```python
from build123d import *

# Parameters (mm, degrees)
CROQUIS2_W              = 135
CROQUIS2_H              = 90
CROQUIS2_R              = 6
SALIENTE_EXTRUIR1_DEPTH = 10
CROQUIS3_W              = 75
CROQUIS3_H              = 90
SALIENTE_EXTRUIR2_DEPTH = 10
CROQUIS4_W              = 55
CROQUIS4_H              = 20
CORTAR_EXTRUIR1_DEPTH   = 91
SALIENTE_EXTRUIR3_DEPTH = 6
CROQUIS11_R             = 10
SALIENTE_EXTRUIR4_DEPTH = 37.5
SALIENTE_EXTRUIR5_DEPTH = 3


with BuildPart() as part:
    # Croquis2 → Saliente-Extruir1 (new body)
    with BuildSketch(Plane(origin=(0, 0, 0), x_dir=(1, 0, 0), z_dir=(0, 1, 0))):
        Rectangle(CROQUIS2_W, CROQUIS2_H)
        with Locations((-53, -25)):
            Circle(CROQUIS2_R, mode=Mode.SUBTRACT)
        with Locations((53, -25)):
            Circle(CROQUIS2_R, mode=Mode.SUBTRACT)
        with Locations((53, 25)):
            Circle(CROQUIS2_R, mode=Mode.SUBTRACT)
        with Locations((-53, 25)):
            Circle(CROQUIS2_R, mode=Mode.SUBTRACT)
    extrude(amount=SALIENTE_EXTRUIR1_DEPTH)

    # Croquis3 → Saliente-Extruir2 (add)
    with BuildSketch(Plane(origin=(0, 10, 0), x_dir=(1, 0, 0), z_dir=(0, 1, 0))):
        Rectangle(CROQUIS3_W, CROQUIS3_H)
    extrude(amount=SALIENTE_EXTRUIR2_DEPTH)

    # Croquis4 → Cortar-Extruir1 (cut, through all)
    with BuildSketch(Plane.XY.offset(45)):
        Rectangle(CROQUIS4_W, CROQUIS4_H)
    extrude(amount=-CORTAR_EXTRUIR1_DEPTH, mode=Mode.SUBTRACT)

    # Croquis9 → Saliente-Extruir3 (add)
    with BuildSketch(Plane.XY.offset(8)):
        Polygon((37.5, 20), (37.5, 10), (67.5, 10), align=None)
    saliente_extruir3 = extrude(amount=-SALIENTE_EXTRUIR3_DEPTH)

    # Simetría1: Saliente-Extruir3 across plane
    add(saliente_extruir3.mirror(Plane(origin=(0, 0, 0), x_dir=(0, 0, 1), z_dir=(1, 0, 0))))

    # Croquis11 → Saliente-Extruir4 (add, symmetric)
    with BuildSketch(Plane(origin=(0, 0, 0), x_dir=(0, 0, -1), z_dir=(1, 0, 0))):
        with BuildLine():
            Line((45, 20), (45, 55))
            ThreePointArc((45, 55), (25, 75), (5, 55))
            Line((5, 55), (5, 20))
            Line((5, 20), (45, 20))
        make_face()
        with Locations((25, 55)):
            Circle(CROQUIS11_R, mode=Mode.SUBTRACT)
    extrude(amount=SALIENTE_EXTRUIR4_DEPTH, both=True)

    # Croquis12 → Saliente-Extruir5 (add, symmetric)
    with BuildSketch(Plane(origin=(0, 0, 0), x_dir=(0, 0, -1), z_dir=(1, 0, 0))):
        Polygon((-45, 20), (10.271335942, 68.678995905), (5, 20), align=None)
    extrude(amount=SALIENTE_EXTRUIR5_DEPTH, both=True)


solid = part.part
```
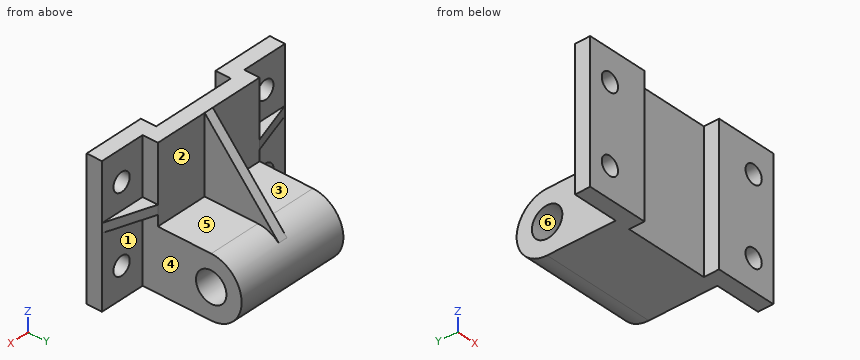
Check sheet for the modelled part. Datum: model origin and axes. Units: mm. Face numbers are marked on the shaded views. A direction names the side the tool comes from. Give positions to 0.01 mm unless a question says otherwise; leave off trailing zeros. Order: outer loops, then holes, each group sorted by start corner. A loop starts at its lowest first (then second) coordinate and runs counter-clockwise, first axis right, second up. Notation, with made-up numbers: (-7.75, 16.5) -> (41.25, 16.5) arc R6 ccw to (41.25, 25.5) -> close; hole circle Ø4 at (21.25, 26). An arc over 180 degrees is marked (long way). Return JSON: item names as keys, results as strings.
1. Set-up check for the marked faces 1, 2 and 3: record each of +Z, -Z, +X, -X, +Y, -Y from which the full face is reachable in a straight line by a thin tool's end or side.
From the geometry:
{"face 1": "-Z, +X, +Y", "face 2": "+Z, +X, +Y", "face 3": "+Z, -X, +Y"}
2. Cross-section at A-A, the plane x = 22.5. Record the cut outline in (y, z).
From the geometry:
{"outline": "(10, -45) -> (55, -45) arc R20 ccw to (55, -5) -> (20, -5) -> (20, 45) -> (10, 45) -> close; hole circle Ø20 at (55, -25)"}
3. Mould release check, pull along Z, two halves, no side actions. Record for the marked faces 4, 5 and 6: +Z half, -Z half, draft (parallel to the pull), parting line (faces both ways), or undercut.
From the geometry:
{"face 4": "draft", "face 5": "+Z half", "face 6": "undercut"}
4. Material ranges on probe 1 along X at (y, z) = (4, -25); probe 2 along Z at (x, y) = (-53, 3); probe 3 along X at (y, z) = (12.5, -27.5), recorded low to high. Write a range as [from, to].
From the geometry:
{"probe 1": "[-67.5, -59], [-47, -27.5], [27.5, 47], [59, 67.5]", "probe 2": "[-45, -31], [-19, 19], [31, 45]", "probe 3": "[-37.5, 37.5]"}
5. Go/stop test with flat-tipped pins: P1, Ø3, axis at x = 6, y = 60.5, coming from the +Z side; P2, Ø9, axis at x = -48.5, z = -26.5, coming from the +Y side; P3, Ø2, axis at x = -10.5, z = 9, coming from the -Y side; P4, Ø12, axis at y = 55, z = -25, coming from the +X side. Record where each tip stops, or that it passes through.
From the geometry:
{"P1": "z = -5.4", "P2": "y = 10", "P3": "y = 10", "P4": "through"}
6. Cross-section at B-B, the plane z = -25. Record the cut outline in (x, y).
From the geometry:
{"outline": "(-67.5, 0) -> (-59, 0) -> (-59, 10) -> (-67.5, 10) -> close; (-47, 0) -> (-27.5, 0) -> (-27.5, 10) -> (27.5, 10) -> (27.5, 0) -> (47, 0) -> (47, 10) -> (37.5, 10) -> (37.5, 45) -> (-37.5, 45) -> (-37.5, 10) -> (-47, 10) -> close; (-37.5, 65) -> (37.5, 65) -> (37.5, 75) -> (-37.5, 75) -> close; (59, 0) -> (67.5, 0) -> (67.5, 10) -> (59, 10) -> close"}
7. Cross-section at D-D, the plane x = -51. Record the cut outline in (y, z).
From the geometry:
{"outline": "(0, -45) -> (10, -45) -> (10, -30.66) -> (0, -30.66) -> close; (0, -19.34) -> (10, -19.34) -> (10, 2) -> (15.5, 2) -> (15.5, 8) -> (10, 8) -> (10, 19.34) -> (0, 19.34) -> close; (0, 30.66) -> (10, 30.66) -> (10, 45) -> (0, 45) -> close"}
8. Cross-section at C-C, the plane y = 63. Record the cut outline in (x, z).
From the geometry:
{"outline": "(-37.5, -43.33) -> (37.5, -43.33) -> (37.5, -31) -> (-37.5, -31) -> close; (-37.5, -19) -> (37.5, -19) -> (37.5, -6.67) -> (3, -6.67) -> (3, -3.82) -> (-3, -3.82) -> (-3, -6.67) -> (-37.5, -6.67) -> close"}
